Drawing for the job (mm, zero at the part's lowest x, y, z). A direction names the side the tool comes from. Round coordinates to 2 decimals unless told otherwise and drop trailing zeros. Loops run counter-clockwise (first coordinate to the right, second up) from the corner with the lowest first, then second, coordinate; pieces in that order, holes last. Notation, with made-up numbers: M 47.5,-36.75 L 86.5,-36.75 A25 ccw 86.5,-15.75 Z; hole C 28,-35 d7. An arc over 180 degrees is marked long. Use a Markdown table: item, result. Add a question column.
Q1. Mould opens along Z. For the marked faces 1, 2 and 3 say: +Z half, -Z half, draft (parallel to the pull), parting line (faces both ways), or undercut.
Q2. Pin check, flat tips, straight feed: pin 1 (1.5 mm diameter, centred on x = 11, y = 5.5, fed in from -Z); pin 2 (2 mm diameter, centred on x = 3.5, y = 5.5, fed in from +Z); pin 3 (2 mm diameter, centred on x = 8.5, y = 2, fed in from +Z). Stop position of each tip, or through.
Q3. Tool access for the marked faces 4, 5 and 6: list every direction of +Z, -Z, +X, -X, +Y, -Y with a clear straight run to the whole face (end or side of a thin tool).
Q4. Cut at B-B (x = 7). Give the cut face in (y, z), plus the area to 3 significant figures.
Q5. Probe line 1 (X direction, y = 0.95, z = 7); line 2 (X direction, y = 8.25, z = 2.5); line 3 (Y direction, x = 12.75, z = 4). List the from-to ranges inside material, lowest first. Write a range as from..to.
Q6. Cut at C-C (y = 4.5). Give the cut face in (x, z), plus the area to 3 significant figures.
Q7. Cut at A-A (z = 7). Give the cut face in (x, y), plus the area to 3 significant figures.
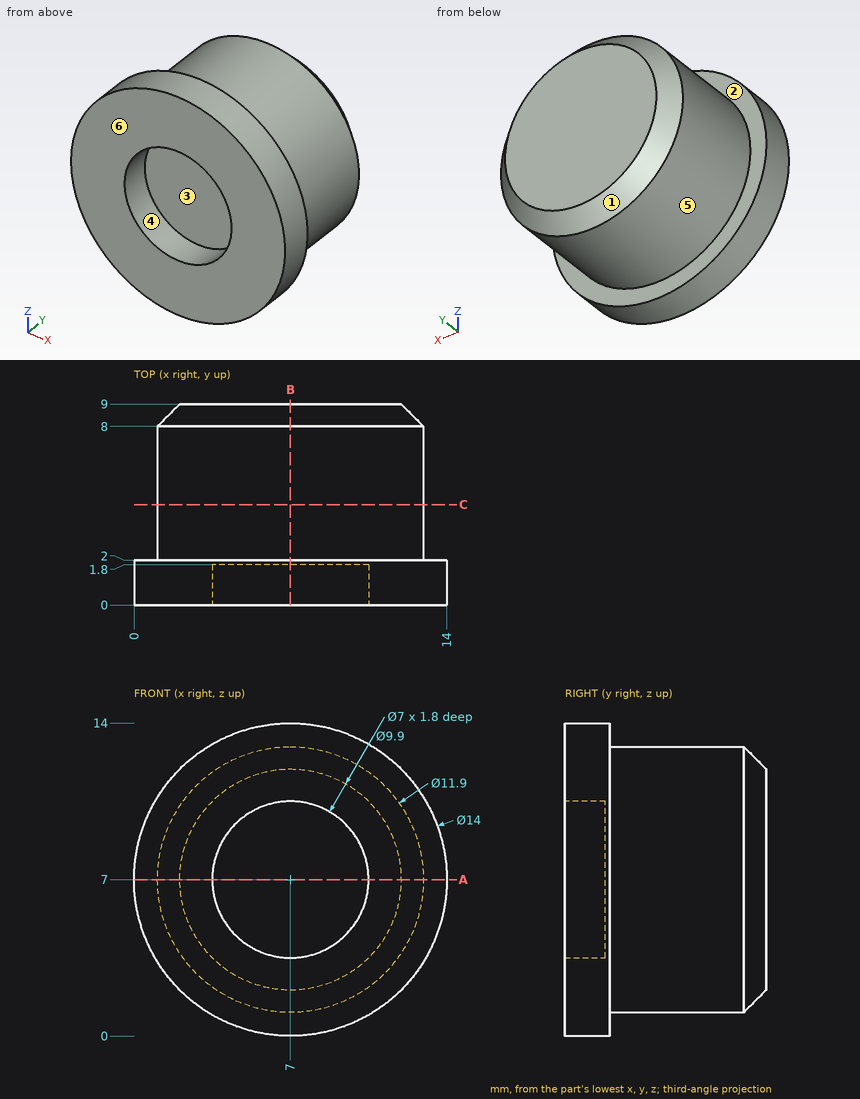
Checked values:
| question | item | result |
|---|---|---|
| 1 | face 1 | parting line |
| 1 | face 2 | draft |
| 1 | face 3 | undercut |
| 2 | pin 1 | stops at z = 2.02 |
| 2 | pin 2 | stops at z = 12.4 |
| 2 | pin 3 | stops at z = 13.98 |
| 3 | face 4 | -Y |
| 3 | face 5 | +Y |
| 3 | face 6 | +Z, -Z, +X, -X, -Y |
| 4 | outline | M 0,0 L 2,0 L 2,1.05 L 8,1.05 L 9,2.05 L 9,11.95 L 8,12.95 L 2,12.95 L 2,14 L 0,14 L 0,10.5 L 1.8,10.5 L 1.8,3.5 L 0,3.5 Z |
| 4 | area | 97.7 mm^2 |
| 5 | line 1 | x = 0..3.5, 10.5..14 |
| 5 | line 2 | x = 3.5..10.5 |
| 5 | line 3 | y = 0..2 |
| 6 | outline | C 7,7 d11.9 |
| 6 | area | 111 mm^2 |
| 7 | outline | M 0,0 L 3.5,0 L 3.5,1.8 L 10.5,1.8 L 10.5,0 L 14,0 L 14,2 L 12.95,2 L 12.95,8 L 11.95,9 L 2.05,9 L 1.05,8 L 1.05,2 L 0,2 Z |
| 7 | area | 97.7 mm^2 |
